from build123d import *

# Parameters (mm, degrees)
F1_DEPTH       = 800
F2_SIZE        = 15
F3_R           = 5
F5_D           = 22
F5_CBORE_D     = 36
F5_CBORE_DEPTH = 23
F6_D           = 22
F6_CBORE_D     = 36
F6_CBORE_DEPTH = 23
F7_D           = 22
F7_CBORE_D     = 36
F7_CBORE_DEPTH = 23


with BuildPart() as f1:
    # F0 (on Front) → F1 (new body)
    with BuildSketch(Plane.XZ):
        Polygon((70, -30), (70, 30), (42.5, 30), (42.5, 6), (-46.5, 6), (-46.5, 30), (-70, 30), (-70, -30), align=None)
    extrude(amount=F1_DEPTH)

    # F2
    f2_edges = [f1.edges().sort_by_distance(p)[0] for p in [
        (-46.5, -400, 30),
        (42.5, -400, 30),
    ]]
    chamfer(f2_edges, length=F2_SIZE)

    # F3
    f3_edges = [f1.edges().sort_by_distance(p)[0] for p in [
        (-61.5, -400, 30),
        (-46.5, -400, 15),
        (-46.5, -400, 6),
        (57.5, -400, 30),
        (42.5, -400, 15),
        (42.5, -400, 6),
        (-70, -400, -30),
        (70, -400, -30),
        (0, -800, -30),
        (0, 0, -30),
    ]]
    fillet(f3_edges, radius=F3_R)

    # F5 (through all)
    with Locations(Plane.XY.offset(6)):
        with Locations((0, -70)):
            CounterBoreHole(F5_D / 2, F5_CBORE_D / 2, F5_CBORE_DEPTH)

    # F6 (through all)
    with Locations(Plane.XY.offset(6)):
        with Locations((0, -400)):
            CounterBoreHole(F6_D / 2, F6_CBORE_D / 2, F6_CBORE_DEPTH)

    # F7 (through all)
    with Locations(Plane.XY.offset(6)):
        with Locations((0, -730)):
            CounterBoreHole(F7_D / 2, F7_CBORE_D / 2, F7_CBORE_DEPTH)


solid = f1.part
Verification items for the finished model (mm, model axes). A direction names the side the tool comes from. Round coordinates to 2 decimals unless told otherwise and drop trailing zeros. Order: outer loops, then holes, each group sorted by start corner. A loop starts at its lowest first (then second) coordinate and runs counter-clockwise, first axis right, second up.
1. Section check B-B on y = -730. Record the cut outline in (x, z).
Final values:
outline: (-70, -25) arc R5 ccw to (-65, -30) - (-11, -30) - (-11, -17) - (-18, -17) - (-18, 6) - (-41.5, 6) arc R5 cw to (-46.5, 11) - (-46.5, 12.93) arc R5 ccw to (-47.96, 16.46) - (-60.04, 28.54) arc R5 ccw to (-63.57, 30) - (-70, 30) - close; (11, -30) - (65, -30) arc R5 ccw to (70, -25) - (70, 30) - (59.57, 30) arc R5 ccw to (56.04, 28.54) - (43.96, 16.46) arc R5 ccw to (42.5, 12.93) - (42.5, 11) arc R5 cw to (37.5, 6) - (18, 6) - (18, -17) - (11, -17) - close
2. Access from +Z, -Z, +X, -X, +Y, -Y to the whole of each face (thin tool, end or side, straight path). Record for faces 1 (the flat face through (-19, -394, 6)), 2 (the flat face through (8, -722, -17)), 3 (the cylindrical face through (2.38, -740.74, -23.59)).
Final values:
face 1: +Z, +Y, -Y
face 2: +Z
face 3: +Z, -Z
3. Section check A-A on z = -6.5. Record the cut outline in (x, y).
Final values:
outline: (-70, -800) - (70, -800) - (70, 0) - (-70, 0) - close; hole circle Ø36 at (0, -730); hole circle Ø36 at (0, -400); hole circle Ø36 at (0, -70)
4. Section check D-D on x = -30. Record the cut outline in (y, z).
Final values:
outline: (-800, -25) arc R5 ccw to (-795, -30) - (-5, -30) arc R5 ccw to (0, -25) - (0, 6) - (-800, 6) - close
5. Release check for a two-part mould opening along X. For faces 4 (the cylindrical face through (-2.343, -52.153, -5.339)), 5 (the flat face through (70, -394, 2)), 6 (the flat face through (-70, -394, 3)) record: +X half, -X half, draft (parallel to the pull), parting line (faces both ways), or undercut.
Final values:
face 4: undercut
face 5: +X half
face 6: -X half
6. Section check C-C on x = 0. State how many separate pieces and enclosed holes the cut face has, then the cut area to 3 significant figures.
Final values:
separate pieces: 4
enclosed holes: 0
area: 25,400 mm2
7. Thickness scan on L1, parallel to Y at x = 0, z = -25.75; L2, parallel to Y at x = 0, z = -24; L3, parallel to X at y = -375.5, z = 11.5. Record the ranges inside material, lowest first.
Final values:
L1: y = -799.94 to -741, -719 to -411, -389 to -81, -59 to -0.06
L2: y = -800 to -741, -719 to -411, -389 to -81, -59 to 0
L3: x = -70 to -46.5, 42.5 to 70
8. Go/stop test with flat-tipped pins: P1, Ø18, axis at x = -1.5, y = -722.5, coming from the +Z side; P2, Ø21.5, axis at x = 0, y = -730, coming from the +Z side; P3, Ø5, axis at x = 3, y = -214, coming from the +Z side. Record where each tip stops, or that it passes through.
Final values:
P1: stops at z = -17
P2: passes through
P3: stops at z = 6
